Source: CAD feature listing. Evaluate the final solid. Frame: model axes, mm. A direction names the side the tool comes from. Give positions to 0.01 mm unless a question says otherwise; leave off trailing zeros. Answer as a JSON object with one key per item and string values. Group by question number.
```python
from build123d import *

# Parameters (mm, degrees)
FILLET1_R            = 2
M4_CLEARANCE_HOLE1_D = 4.5
CIRPATTERN1_COUNT    = 24
SKETCH6_R            = 2.25
SKETCH6_R_2          = 2
BOSS_EXTRUDE1_DEPTH  = 6


with BuildPart() as part:
    # Sweep1: sweep along a path in Sketch1
    with BuildLine(Plane.XY) as sweep1_path:
        CenterArc((0, 0), 216.325, 0, 360)
    # Sketch2 → Sweep1 (sweep)
    with BuildSketch(Plane(origin=(0, 0, 0), x_dir=(0, 0, -1), z_dir=(1, 0, 0))):
        with BuildLine():
            Line((0, 227.325), (0, 219.325))
            ThreePointArc((0, 219.325), (0.878679656, 217.203679656), (3, 216.325))
            Line((3, 216.325), (35, 216.325))
            Line((35, 216.325), (35, 217.39))
            Line((35, 217.39), (3.1, 217.39))
            ThreePointArc((3.1, 217.39), (1.685786438, 217.975786438), (1.1, 219.39))
            Line((1.1, 219.39), (1.1, 227.325))
            Line((1.1, 227.325), (0, 227.325))
        make_face()
    sweep(path=sweep1_path.line)

    # Sketch7 → Revolve3 (revolve)
    with BuildSketch(Plane(origin=(0, 0, 0), x_dir=(0, 0, -1), z_dir=(1, 0, 0)), mode=Mode.PRIVATE) as revolve3_sk:
        with BuildLine():
            Line((6, 216.325), (3, 216.325))
            ThreePointArc((3, 216.325), (0.878679656, 217.203679656), (0, 219.325))
            Line((0, 219.325), (0, 227.325))
            Line((0, 227.325), (6, 227.325))
            Line((6, 227.325), (6, 216.325))
        make_face()
    revolve(revolve3_sk.sketch.rotate(Axis((0, 0, 0), (0, 0, -1)), 270), axis=Axis((0, 0, 0), (0, 0, -1)))  # turned: the seam where the file's is

    # Fillet1
    fillet1_edges = [part.edges().sort_by_distance(p)[0] for p in [
        (-217.39, 0, -6),
    ]]
    fillet(fillet1_edges, radius=FILLET1_R)

    # Sketch8 → Cut-Revolve1 (revolve, cut)
    with BuildSketch(Plane(origin=(0, 0, 0), x_dir=(0, 0, -1), z_dir=(1, 0, 0)), mode=Mode.PRIVATE) as cut_revolve1_sk:
        Polygon((35, 216.751), (28.40975, 216.751), (28.19675, 216.964), (21.6065, 216.964), (21.3935, 217.177), (14.80325, 217.177), (14.59025, 217.39), (35, 217.39), align=None)
    revolve(cut_revolve1_sk.sketch.rotate(Axis((0, 0, -21), (0, 0, 1)), 90), axis=Axis((0, 0, -21), (0, 0, 1)), mode=Mode.SUBTRACT)  # turned: the seam where the file's is

    # M4 Clearance Hole1 (through all)
    with Locations(Plane.XY):
        with Locations((0, 222)):
            m4_clearance_hole1 = Hole(M4_CLEARANCE_HOLE1_D / 2)

    # CirPattern1: M4 Clearance Hole1 ×24 about axis
    cirpattern1_axis = Axis((0, 0, 0), (0, 0, 1))
    for i in range(1, CIRPATTERN1_COUNT):
        add(m4_clearance_hole1.rotate(cirpattern1_axis, i * 360 / CIRPATTERN1_COUNT), mode=Mode.SUBTRACT)

    # Sketch6 → Boss-Extrude1 (add)
    with BuildSketch(Plane.XY):
        with Locations((-222, 0)):
            Circle(SKETCH6_R)
        with Locations((-222, 0)):
            Circle(SKETCH6_R_2, mode=Mode.SUBTRACT)
        with Locations((222, 0)):
            Circle(SKETCH6_R)
        with Locations((222, 0)):
            Circle(SKETCH6_R_2, mode=Mode.SUBTRACT)
    extrude(amount=-BOSS_EXTRUDE1_DEPTH)


solid = part.part
```
(1) Ray query, L1, parallel to Y at x = 0, z = -4.5 (3 decimals); L2, parallel to X at y = -3.5, z = -29; L3, parallel to X at y = -111, z = -3.25. Return the intervals inside material, ascending. Write a range as [from, to].
(2) Pull-direction query (X, two-part tool) for faces 1 (the flat face through (-119, 186, -6)), 2 (the cylindrical face through (206.336, 64.978, -19.224)), 3 (the cylindrical face through (207.35, 65.3, -11.25)); classes: pulls with the +X half, pulls with the -X half, needs draft (parallel to the pull), parting line crosses it, or undercut.
(3) Contact query for flat-ended pins moving along their axis: pin 1 Ø8 at (y, z) = (80, -9) entering from +X; pin 2 Ø4 at (x, y) = (-192.26, 111) entering from +Z; pin 3 Ø8 at (x, y) = (-144.5, -167) entering from -Z; pin 4 Ø5 at (x, y) = (0, 222) entering from -Z. Output: stop coordinate, or through.
(4) Access query for faces 4 (the cylindrical face through (-100.017, 192.295, -31.659)), 5 (the flat face through (-119, 186, 0)). Directions: +Z, -Z, +X, -X, +Y, -Y. A direction counts if a zero-diameter tool reaches every point of the face in a straight line with its end or side. Return the directions, or none.
Reported:
{
 "1": {"L1": "y = [-227.325, -224.25], [-219.75, -216.325], [216.325, 219.75], [224.25, 227.325]", "L2": "x = [-216.72, -216.3], [216.3, 216.72]", "L3": "x = [-198.38, -194.51], [-190.01, -185.68], [185.68, 190.01], [194.51, 198.38]"},
 "2": {"face 1": "needs draft", "face 2": "undercut", "face 3": "parting line crosses it"},
 "3": {"pin 1": "stops at x = 213.76", "pin 2": "passes through", "pin 3": "stops at z = -28.32", "pin 4": "stops at z = -6"},
 "4": {"face 4": "-Z", "face 5": "+Z, +X, -X, +Y, -Y"}
}
